Autodesk Inventor part; units mm, degrees
ref_plane "YZ Plane" through (0, 0, 0) normal (1, 0, 0) x (0, 1, 0)
ref_plane "XZ Plane" through (0, 0, 0) normal (0, 1, 0) x (-1, 0, 0)
ref_plane "XY Plane" through (0, 0, 0) normal (0, 0, 1) x (1, 0, 0)
sketch "Sketch1" plane through (0, 0, 0) normal (0, 1, 0) x (-1, 0, 0)
  circle A0 centre (0, 0) radius 1.5
  dimension "d0" = 3
extrude "Extrusion1" add sketch "Sketch1" along normal blind 6
sketch "Sketch2" plane through (0, 6, 0) normal (0, 1, 0) x (1, 0, 0)
  circle A0 centre (0, 0) radius 1.5
  circle A1 centre (0, 0) radius 2.75
  dimension "d3" = 5.5
extrude "Extrusion2" add sketch "Sketch2" along normal blind 3 contours A0 | A1
sketch "Sketch3" plane through (0, 9, 0) normal (0, 1, 0) x (1, 0, 0)
  circle A0 centre (0, 0) radius 2.75
  line L0 (0, 1.4434) -> (1.25, 0.7217)
  line L1 (1.25, 0.7217) -> (1.25, -0.7217)
  line L2 (1.25, -0.7217) -> (0, -1.4434)
  line L3 (0, -1.4434) -> (-1.25, -0.7217)
  line L4 (-1.25, -0.7217) -> (-1.25, 0.7217)
  line L5 (-1.25, 0.7217) -> (0, 1.4434)
  dimension "d6" = 2.5
extrude "Extrusion3" cut sketch "Sketch3" against normal blind 2 contours L0 L1 L2 L3 L4 L5
thread "Thread1"
chamfer "Chamfer1" distance 0.5 angle 45 1 edges at (1.5, 0, 0)
properties part number "SHCS3x6" material "Stainless Steel"
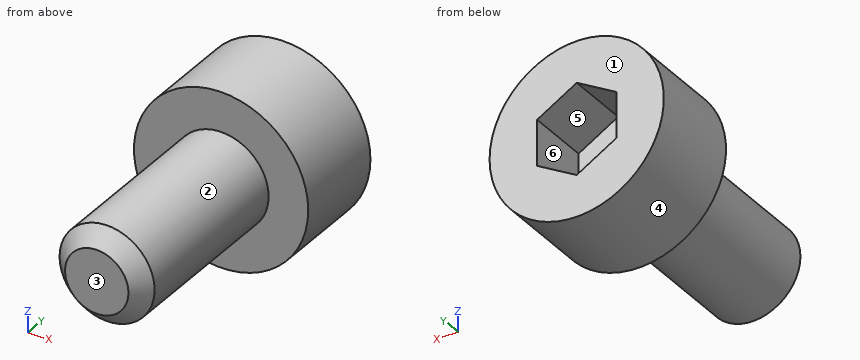
Geometry: final body of the model. Coordinates: model frame, mm. Face numbers are marked on the shaded views. A direction names the side the tool comes from. Give positions to 0.01 mm unless a question says otherwise; leave off trailing zeros. Loops run counter-clockwise (first coordinate to the right, second up) from the corner with the lowest first, then second, coordinate; pieces in that order, holes last. Notation, with made-up numbers: M 7,25.25 L 52,25.25 A21 cw 52,41.25 Z; hole C 60,-23 d2. An arc over 180 degrees is marked long. Put each result on its own line as item: value.
1) Cut plane B-B, the plane z = 0. Return the cut outline in (x, y), plus the area to 4 significant figures.
Computed values:
outline: M -2.75,6 L -1.5,6 L -1.5,0.5 L -1,0 L 1,0 L 1.5,0.5 L 1.5,6 L 2.75,6 L 2.75,9 L 1.25,9 L 1.25,7 L -1.25,7 L -1.25,9 L -2.75,9 Z
area: 29.25 mm^2
2) Cut plane A-A, the plane y = 7.75. Return the cut outline in (x, z), plus the area to 3 significant figures.
Computed values:
outline: C 0,0 d5.5; hole M -1.25,-0.72 L 0,-1.44 L 1.25,-0.72 L 1.25,0.72 L 0,1.44 L -1.25,0.72 Z
area: 18.3 mm^2
3) Cut plane D-D, the plane x = -1.9. Return the cut outline in (y, z).
Computed values:
outline: M 6,-1.99 L 9,-1.99 L 9,1.99 L 6,1.99 Z
4) Material intervals for L1, parallel to Y at x = 1.4, z = -2.3; L2, parallel to Y at x = 0.15, z = -0.3; L3, parallel to Z at x = -1.25, y = 4.5, sorted ascending. Write a range as from..to.
Computed values:
L1: y = 6..9
L2: y = 0..7
L3: z = -0.83..0.83
5) Reachability of the marked faces 1 and 2 from +Z, -Z, +X, -X, +Y, -Y: full face, straight path, thin tool, end or side. Return the list, or none.
Computed values:
face 1: +Z, -Z, +X, -X, +Y
face 2: -Y
6) First-contact query: P1, Ø3, axis at y = 3.5, z = 1, coming from the +X side. Flat tip, straight axial feed; report the tip coordinate or a pass-through.
Computed values:
P1: stops at x = 1.5
7) Cut plane C-C, the plane y = 5.75. Return the cut outline in (x, z), plus the area to 3 significant figures.
Computed values:
outline: C 0,0 d3
area: 7.07 mm^2
8) Mould query, pull axis X, two halves, no side actions, for the marked faces 3, 4, 5 and 6. Classes: released by +X, released by -X, zero draft, split by the parting line, or undercut.
Computed values:
face 3: zero draft
face 4: split by the parting line
face 5: undercut
face 6: undercut
